from build123d import *

# Parameters (mm, degrees)
F1_DEPTH = 50
F3_DEPTH = 0.6
F4_R     = 0.5
F5_DEPTH = 1


with BuildPart() as f1:
    # F0 (on Front) → F1 (new body)
    with BuildSketch(Plane.XZ):
        Polygon((45.7524405147, 0), (45.7524405147, 3), (5.7524405147, 3), (30.5011778563, 27.7487373415), (28.3798575127, 29.8700576851), (2.7524405147, 4.2426406871), (2.7524405147, 0), align=None)
    extrude(amount=F1_DEPTH)

    # F2 (on face) → F3 (join)
    with BuildSketch(Plane(origin=(-0.7451000862, 0, 0.7451000862), x_dir=(0, -1, 0), z_dir=(-0.7071067812, 0, 0.7071067812))):
        Polygon((28.6160509516, 19.0431820663), (26.9152817478, 20.0955052655), (17.1134265816, 32.7415969661), (10, 27.2280534351), (19.8018551662, 14.5819617345), (20.3959014762, 12.672221181), (21.9274413459, 10.6962693528), (31.8867334894, 4.9462693528), (39.542422512, 4.9462693528), align=None)
        with BuildLine():
            ThreePointArc((16.2533213032, 24.546920712), (16.4666390433, 26.230516727), (18.1502350583, 26.0171989869))
            Line((18.1502350583, 26.0171989869), (20.4781756603, 23.013752208))
            ThreePointArc((20.4781756603, 23.013752208), (20.6650927856, 22.6671048639), (20.7297187827, 22.2786130705))
            ThreePointArc((20.7297187827, 22.2786130705), (19.918210576, 21.1432390676), (18.5812619052, 21.5434739331))
            Line((18.5812619052, 21.5434739331), (16.2533213032, 24.546920712))
        make_face(mode=Mode.SUBTRACT)
        Polygon((45.74313995, -3.0537306472), (39.542422512, 4.9462693528), (31.8867334894, 4.9462693528), align=None)
    extrude(amount=F3_DEPTH)

    # F4
    f4_edges = [f1.edges().sort_by_distance(p)[0] for p in [
        (22.194573, -17.113427, 24.109037),
        (18.295909, -10, 20.210373),
    ]]
    fillet(f4_edges, radius=F4_R)

    # F2 (on face) → F5 (join, symmetric)
    with BuildSketch(Plane(origin=(-0.7451000862, 0, 0.7451000862), x_dir=(0, -1, 0), z_dir=(-0.7071067812, 0, 0.7071067812))):
        with BuildLine():
            ThreePointArc((18.1502350583, 26.0171989869), (18.3371521837, 25.6705516428), (18.4017781807, 25.2820598494))
            ThreePointArc((18.4017781807, 25.2820598494), (17.590269974, 24.1466858465), (16.2533213032, 24.546920712))
            Line((16.2533213032, 24.546920712), (18.5812619052, 21.5434739331))
            ThreePointArc((18.5812619052, 21.5434739331), (18.7945796452, 23.2270699481), (20.4781756603, 23.013752208))
            Line((20.4781756603, 23.013752208), (18.1502350583, 26.0171989869))
        make_face()
        with BuildLine():
            ThreePointArc((16.2533213032, 24.546920712), (17.590269974, 24.1466858465), (18.4017781807, 25.2820598494))
            ThreePointArc((18.4017781807, 25.2820598494), (18.3371521837, 25.6705516428), (18.1502350583, 26.0171989869))
            ThreePointArc((18.1502350583, 26.0171989869), (16.4666390433, 26.230516727), (16.2533213032, 24.546920712))
        make_face()
        with BuildLine():
            ThreePointArc((20.7297187827, 22.2786130705), (20.6650927856, 22.6671048639), (20.4781756603, 23.013752208))
            ThreePointArc((20.4781756603, 23.013752208), (18.7945796452, 23.2270699481), (18.5812619052, 21.5434739331))
            ThreePointArc((18.5812619052, 21.5434739331), (19.918210576, 21.1432390676), (20.7297187827, 22.2786130705))
        make_face()
    extrude(amount=F5_DEPTH, both=True)


solid = f1.part
Verification items for the finished model (mm, model axes). A direction names the side the tool comes from. Give positions to 0.01 mm unless a question says otherwise; leave off trailing zeros. Loops run counter-clockwise (first coordinate to the right, second up) from the corner with the lowest first, then second, coordinate; pieces in that order, holes last. Notation, with made-up numbers: (61, -25.75) - (76, -25.75) arc R9 ccw to (76, -10.75) - close; hole circle Ø5 at (71, 61). An arc over 180 degrees is marked (long way). Write each question's results on one line, items separated by ' | '.
1) Depth check by flat-ended pin: P1, Ø12, axis at y = -26, z = 20.5, coming from the -X side; P2, Ø1.5, axis at y = -39.5, z = 15, coming from the -X side; P3, Ø12, axis at x = 6, y = -29.5, coming from the +Z side (3 decimals). Enter the tip coordinate at first touch or a pass-through.
Solution:
P1: x = 12.16 | P2: x = 12.76 | P3: z = 14.315
2) Sectioned sample at B-B on y = -7. Record the boundary of the cut face in (x, z), plus the area to 3 significant figures.
Solution:
outline: (2.75, 0) - (45.75, 0) - (45.75, 3) - (5.75, 3) - (30.5, 27.75) - (28.38, 29.87) - (2.75, 4.24) - close | area: 238 mm2
3) Sectioned sample at D-D on z = 13. Record the boundary of the cut face in (x, y).
Solution:
outline: (10.66, -30.41) - (11.51, -29.94) - (11.51, -50) - (15.75, -50) - (15.75, 0) - (11.51, 0) - (11.51, -17.67) - (10.66, -18.14) - close
4) Material ranges on L1, parallel to Z at x = 25.5, y = -2; L2, parallel to Z at x = 42, y = -24; L3, parallel to Z at x = 11.5, y = -20, recorded low to high. Write a range as from..to.
Solution:
L1: 0..3, 22.75..26.99 | L2: 0..3 | L3: 0..3, 8.75..13.84
5) Tool access check on faces 1 (the flat face through (17.95, -24.65, 15.2)), 2 (the flat face through (8.691, -20.095, 10.6)), 3 (the flat face through (0.98, -38.78, 2.47)), 4 (the flat face through (16.01, -19.33, 18.63)). Record the directions out of +Z, -Z, +X, -X, +Y, -Y that give a thin tool (end or side, any length) a straight path to the whole face; none if there is none.
Solution:
face 1: +X, +Y, -Y | face 2: -X, +Y | face 3: -Z, +Y, -Y | face 4: +Z, -Y
6) Mould release check, pull along X, two halves, no side actions. Record for faces 5 (the flat face through (17.526, -22.234, 19.435)), 6 (the flat face through (15, -17.4, 17.62)), 7 (the flat face through (45.752, -25, 1)), 8 (the flat face through (21, -50, 2.8)): pulls with the +X half, pulls with the -X half, needs draft (parallel to the pull), parting line crosses it, or undercut.
Solution:
face 5: undercut | face 6: pulls with the -X half | face 7: pulls with the +X half | face 8: needs draft
7) Sectioned sample at C-C on x = 33.5. Record the boundary of the cut face in (y, z).
Solution:
outline: (-50, 0) - (0, 0) - (0, 3) - (-50, 3) - close
8) Sectioned sample at A-A on x = 20.5. Record the boundary of the cut face in (y, z), plus the area to 3 significant figures.
Solution:
outline: (-50, 0) - (0, 0) - (0, 3) - (-50, 3) - close; (-50, 17.75) - (0, 17.75) - (0, 21.99) - (-13.63, 21.99) - (-14.41, 22.84) - (-18.74, 22.84) - (-19.2, 21.99) - (-50, 21.99) - close | area: 366 mm2
